CAD build for the part. Positions are in the model's coordinates, mm. Give positions to 0.01 mm unless a question says otherwise; leave off trailing zeros. Order: outer loops, then holes, each group sorted by start corner. A loop starts at its lowest first (then second) coordinate and runs counter-clockwise, first axis right, second up. Notation, with made-up numbers: M 40.25,44 L 69.25,44 A12 ccw 69.25,48 Z; hole C 19,79.5 d2. An arc over 180 degrees is marked long. Put each result on its own line as item: value. Start each with the question number.
1) Pin check, flat tips, straight feed: pin 1 (3 mm diameter, centred on x = -185.5, z = 8, fed in from -Y); pin 2 (1.1 mm diameter, centred on x = -186, y = 142, fed in from -Z); pin 3 (3 mm diameter, centred on y = 148, z = 5.5, fed in from -X); pin 4 (1 mm diameter, centred on x = -179, z = 5.5, fed in from +Y). Stop position of each tip, or through.
2) Cut at C-C (y = 143.5). Write the cut outline in (x, z), and give its area (3 significant figures).
3) Drill centre lines: line 1 (Z direction, x = -181.5, y = 147); line 2 (Z direction, x = -181.5, y = 147.5); line 3 (Y direction, x = -182, z = 6). Where is each one in solid material? Low to high. Write a range as [from, to].
4) Cut at B-B (z = 3.5). Write the cut outline in (x, y), and give its area (3 significant figures).
5) Cut at D-D (x = -181.75). Write the cut outline in (y, z).
6) Cut at A-A (x = -183). Write the cut outline in (y, z).
```python
from build123d import *

# Parameters (mm, degrees)
BOX235_W                  = 0.5
BOX235_H                  = 1
BOX235_DEPTH              = 15
BOX235_ROLL_ANGLE         = 46
BOX236_W                  = 0.5
BOX236_H                  = 1
BOX236_DEPTH              = 15
BOX236_ROLL_ANGLE         = -46
BOX234_W                  = 0.5
BOX234_H                  = 1
BOX234_DEPTH              = 11
FUSION021_PLACEMENT_ANGLE = -38


with BuildPart() as cubo235:
    # Box235 → Box235 (new body)
    with BuildSketch(Plane.XY):
        with Locations((0.25, 0.5)):
            Rectangle(BOX235_W, BOX235_H)
    extrude(amount=BOX235_DEPTH)


with BuildPart() as cubo235_1:
    # Box235 roll: moved
    add(cubo235.part.rotate(Axis((0, 0, 0), (1, 0, 0)), BOX235_ROLL_ANGLE))


with BuildPart() as cubo235_2:
    # Box235 placement: moved
    add(cubo235_1.part.moved(Location((0, 11, 0.5))))


with BuildPart() as cubo236:
    # Box236 → Box236 (new body)
    with BuildSketch(Plane.XY):
        with Locations((0.25, 0.5)):
            Rectangle(BOX236_W, BOX236_H)
    extrude(amount=BOX236_DEPTH)


with BuildPart() as cubo236_1:
    # Box236 roll: moved
    add(cubo236.part.rotate(Axis((0, 0, 0), (1, 0, 0)), BOX236_ROLL_ANGLE))


with BuildPart() as cubo236_2:
    # Box236 placement: moved
    add(cubo236_1.part.moved(Location((0, 0.4, 1.1))))


with BuildPart() as fusion021:
    # Box234 → Box234 (new body)
    with BuildSketch(Plane.XY.offset(0.5)):
        with Locations((0.25, 0.5)):
            Rectangle(BOX234_W, BOX234_H)
    extrude(amount=BOX234_DEPTH)

    # Fusion021: union Cubo235, Cubo236
    add(cubo235_2.part)
    add(cubo236_2.part)


with BuildPart() as fusion021_1:
    # Fusion021 placement: moved
    add(fusion021.part.moved(Location((-186.16, 141.7, 0))).rotate(Axis((-186.16, 141.7, 0), (0, 0, 1)), FUSION021_PLACEMENT_ANGLE))


solid = fusion021_1.part
```
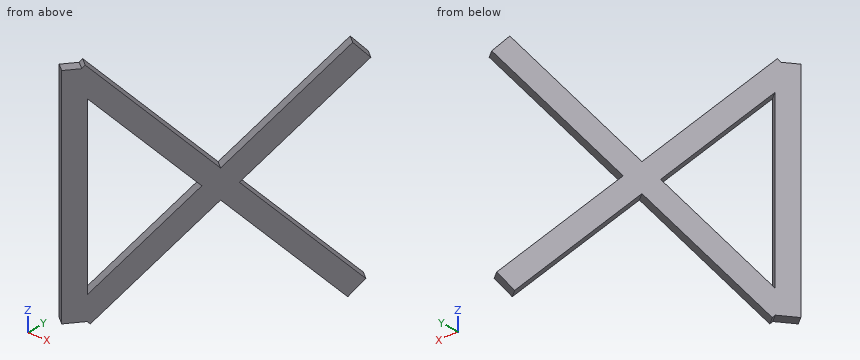
Solution:
1. pin 1: y = 141.39
1. pin 2: z = 0.5
1. pin 3: x = -182.41
1. pin 4: through
2. outline: M -184.75,1.53 L -184.12,1.91 L -184.12,3.3 L -184.75,2.92 Z; M -184.75,8.92 L -184.12,8.54 L -184.12,9.93 L -184.75,10.31 Z
2. area: 1.76 mm²
3. line 1: [4.32, 5.71], [6.13, 7.52]
3. line 2: [3.94, 5.33], [6.51, 7.9]
3. line 3: [146.21, 147.02]
4. outline: M -186.16,141.7 L -185.77,141.39 L -185.15,142.18 L -185.54,142.49 Z; M -184.38,143.97 L -183.99,143.67 L -183.1,144.8 L -183.5,145.11 Z; M -181.3,147.92 L -180.91,147.61 L -180.02,148.75 L -180.41,149.05 Z
4. area: 1.94 mm²
5. outline: M 146.53,4.82 L 147.34,4.21 L 147.34,5.6 L 146.92,5.92 L 147.34,6.24 L 147.34,7.63 L 146.53,7.01 Z
6. outline: M 144.93,3.66 L 145.74,4.28 L 145.74,5.67 L 144.93,5.05 Z; M 144.93,6.78 L 145.74,6.17 L 145.74,7.56 L 144.93,8.17 Z
